Autodesk Inventor part; units mm, degrees
ref_plane "hh_XY" through (0, 3.175, 0) normal (0, 0, 1) x (1, 0, 0)
ref_plane "hh_YZ" through (0, 3.175, 0) normal (1, 0, 0) x (0, 1, 0)
ref_plane "hh_ZX" through (0, 3.175, 0) normal (0, 1, 0) x (0, 0, 1)
sketch "Sketch_1" plane through (0, 0, 0) normal (0, 0, 1) x (1, 0, 0)
  line L0 (6.35, 0) -> (0, 0)
  line L1 (0, 0) -> (0, 2.634)
  line L2 (0, 2.634) -> (0.541, 3.175)
  line L3 (0.541, 3.175) -> (6.35, 3.175)
  line L4 (6.35, 3.175) -> (6.35, 0)
  line L5 (6.35, 0) -> (0, 0)
revolve "Revolution1" add sketch "Sketch_1" angle 360 about axis through (6.35, 0, 0) along (1, 0, 0)
thread "Thread1"
sketch "Sketch_3" plane through (0, 0, 0) normal (0, 0, 1) x (1, 0, 0)
  line L0 (13.2715, 0) -> (6.35, 0)
  line L1 (6.35, 0) -> (6.35, 4.0513)
  line L2 (6.35, 4.0513) -> (6.858, 4.5593)
  line L3 (6.858, 4.5593) -> (9.398, 4.5593)
  line L4 (9.398, 4.5593) -> (9.398, 3.5242)
  line L5 (9.398, 3.5242) -> (9.9568, 3.5242)
  line L6 (9.9568, 3.5242) -> (10.5156, 4.0831)
  line L7 (10.5156, 4.0831) -> (12.7635, 4.0831)
  line L8 (12.7635, 4.0831) -> (13.2715, 3.5751)
  line L9 (13.2715, 3.5751) -> (13.2715, 0)
  line L10 (13.2715, 0) -> (6.35, 0)
revolve "Revolution2" add sketch "Sketch_3" angle 360 about axis through (13.2715, 0, 0) along (1, 0, 0)
sketch "Sketch_4" plane through (0, 0, 0) normal (0, 0, 1) x (1, 0, 0)
  line L0 (15.875, 0) -> (13.2715, 0)
  line L1 (13.2715, 0) -> (13.2715, 2.9845)
  line L2 (13.2715, 2.9845) -> (15.367, 2.9845)
  line L3 (15.367, 2.9845) -> (15.875, 2.4765)
  line L4 (15.875, 2.4765) -> (15.875, 0)
  line L5 (15.875, 0) -> (13.2715, 0)
revolve "Revolution3" add sketch "Sketch_4" angle 360 about axis through (15.875, 0, 0) along (1, 0, 0)
sketch "Sketch4" plane through (0, 0, 0) normal (-1, 0, 0) x (0, 0, 1)
  point P0 (0, 0)
hole "Hole1" at (0, 0, 0) direction (1, 0, 0) diameter 3.2512 depth 15.875 countersink diameter 4.0132 countersink angle 90
sketch "Sketch_47" plane through (0, 0, 0) normal (0, 0, 1) x (1, 0, 0)
  line L0 (9.9568, 0) -> (9.398, 0)
  line L1 (9.398, 4.0431) -> (9.398, 3.2702)
  line L2 (9.398, 3.2702) -> (9.9568, 3.2702)
  line L3 (9.9568, 3.2702) -> (9.9568, 3.5242)
  line L4 (9.9568, 3.5242) -> (9.6774, 3.5242)
  line L5 (9.6774, 3.5242) -> (9.5118, 3.6899)
  arc A0 (9.5118, 3.8695) -> (9.5118, 3.6899) centre (9.6016, 3.7797) ccw
  line L6 (9.5118, 3.8695) -> (10.1174, 4.4751)
  line L7 (10.1174, 4.4751) -> (10.1174, 4.5593)
  line L8 (10.1174, 4.5593) -> (9.9142, 4.5593)
  line L9 (9.9142, 4.5593) -> (9.398, 4.0431)
revolve "Revolution4" add sketch "Sketch_47" angle 360 about axis through (9.9568, 0, 0) along (1, 0, 0)
ref_plane "hh_XY" through (0, 3.175, 0) normal (0, 0, 1) x (1, 0, 0)
ref_plane "hh_YZ" through (0, 3.175, 0) normal (1, 0, 0) x (0, 1, 0)
ref_plane "hh_ZX" through (0, 3.175, 0) normal (0, 1, 0) x (0, 0, 1)
ref_plane "rod_guide_XY" through (0, 0, 0) normal (1, 0, 0) x (0, 0, -1)
ref_plane "rod_guide_YZ" through (0, 0, 0) normal (0, 0, -1) x (0, 1, 0)
ref_plane "rod_guide_ZX" through (0, 0, 0) normal (0, 1, 0) x (1, 0, 0)
ref_plane "t1_XY" through (6.35, 0, 0) normal (1, 0, 0) x (0, 0, -1)
ref_plane "t1_YZ" through (6.35, 0, 0) normal (0, 0, -1) x (0, 1, 0)
ref_plane "t1_ZX" through (6.35, 0, 0) normal (0, 1, 0) x (1, 0, 0)
ref_plane "t111_XY" through (6.35, 0, 0) normal (1, 0, 0) x (0, 0, -1)
ref_plane "t111_YZ" through (6.35, 0, 0) normal (0, 0, -1) x (0, 1, 0)
ref_plane "t111_ZX" through (6.35, 0, 0) normal (0, 1, 0) x (1, 0, 0)
ref_plane "to_foot_bracket_XY" through (6.35, 0, 0) normal (1, 0, 0) x (0, 0, -1)
ref_plane "to_foot_bracket_YZ" through (6.35, 0, 0) normal (0, 0, -1) x (0, 1, 0)
ref_plane "to_foot_bracket_ZX" through (6.35, 0, 0) normal (0, 1, 0) x (1, 0, 0)
ref_plane "to_nut_XY" through (6.35, 0, 0) normal (1, 0, 0) x (0, 0, -1)
ref_plane "to_nut_YZ" through (6.35, 0, 0) normal (0, 0, -1) x (0, 1, 0)
ref_plane "to_nut_ZX" through (6.35, 0, 0) normal (0, 1, 0) x (1, 0, 0)
ref_plane "to_rod_XY" through (0, 0, 0) normal (1, 0, 0) x (0, 0, -1)
ref_plane "to_rod_YZ" through (0, 0, 0) normal (0, 0, -1) x (0, 1, 0)
ref_plane "to_rod_ZX" through (0, 0, 0) normal (0, 1, 0) x (1, 0, 0)
ref_plane "to_screw_XY" through (6.35, 0, 0) normal (0, 1, 0) x (1, 0, 0)
ref_plane "to_screw_YZ" through (6.35, 0, 0) normal (1, 0, 0) x (0, 0, -1)
ref_plane "to_screw_ZX" through (6.35, 0, 0) normal (0, 0, -1) x (0, 1, 0)
ref_plane "to_trunnion_brackets_XY" through (0, 0, 0) normal (0, 1, 0) x (1, 0, 0)
ref_plane "to_trunnion_brackets_YZ" through (0, 0, 0) normal (1, 0, 0) x (0, 0, -1)
ref_plane "to_trunnion_brackets_ZX" through (0, 0, 0) normal (0, 0, -1) x (0, 1, 0)
ref_plane "to_trunnion_brackets1_XY" through (0, 6.35, 0) normal (0, 1, 0) x (1, 0, 0)
ref_plane "to_trunnion_brackets1_YZ" through (0, 6.35, 0) normal (1, 0, 0) x (0, 0, -1)
ref_plane "to_trunnion_brackets1_ZX" through (0, 6.35, 0) normal (0, 0, -1) x (0, 1, 0)
ref_plane "to_trunnion_brackets2_XY" through (0, -6.35, 0) normal (0, 1, 0) x (1, 0, 0)
ref_plane "to_trunnion_brackets2_YZ" through (0, -6.35, 0) normal (1, 0, 0) x (0, 0, -1)
ref_plane "to_trunnion_brackets2_ZX" through (0, -6.35, 0) normal (0, 0, -1) x (0, 1, 0)
ref_plane "to_tube_XY" through (9.9568, 0, 0) normal (1, 0, 0) x (0, 0, -1)
ref_plane "to_tube_YZ" through (9.9568, 0, 0) normal (0, 0, -1) x (0, 1, 0)
ref_plane "to_tube_ZX" through (9.9568, 0, 0) normal (0, 1, 0) x (1, 0, 0)
properties part number "007000-0_rod_guide"
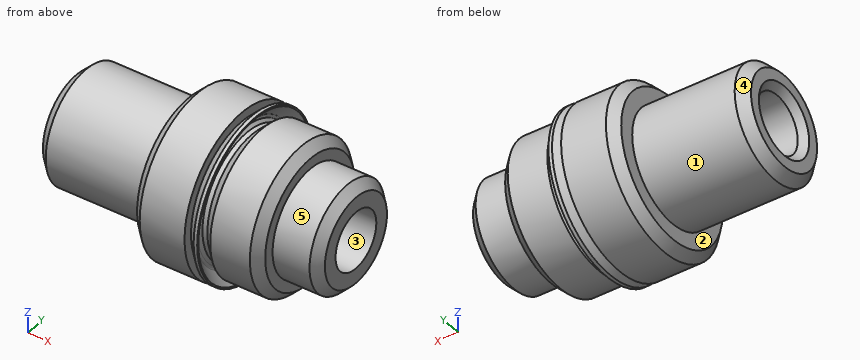
The model under review builds one solid part; all positions refer to its coordinate system, in mm. Face numbers are marked on the shaded views. A direction names the side the tool comes from. Give positions to 0.01 mm unless a question says otherwise; leave off trailing zeros. Write each loop counter-clockwise with the first axis right and the second up, starting at its lowest first coordinate (ties: lowest second). Pieces come first, ordered by that corner, then holes.
1. Tool access review of the marked faces 4 and 5: name each direction out of +Z, -Z, +X, -X, +Y, -Y from which nothing blocks a thin tool from reaching the whole face with its end or side.
2. Wall thickness on L1, parallel to X at y = 2, z = -2.75; L2, parallel to Y at x = 9.75, z = 1; L3, parallel to Z at x = 14, y = -0.75: over which ranges is each line inside the solid? List them lowest first.
3. For P1, Ø2, axis at y = 0, z = 0, coming from the +X side; P2, Ø3, axis at x = 4.5, z = 3, coming from the +Y side; P3, Ø1, axis at x = 14, z = 2.5, coming from the -Y side; P4, Ø1, axis at y = -0.5, z = 3, coming from the +X side, all flat-tipped, find the tip position at first contact; note any pin that passes through.
4. Draft analysis for pull direction Z (two halves, no side actions). For the marked faces 1, 2 and 3, state which applies: +Z half, -Z half, draft (parallel to the pull), parting line (faces both ways), or undercut.
5. Add section A-A, the plane x = 2.5. Write out the cut boundary in (y, z) (3 decimals), plus the area to 3 significant figures.
Worked answers:
1. face 4: -X
1. face 5: +X
2. L1: x = 6.35 to 13.27
2. L2: y = -4.28 to -3.98, -3.38 to -1.28, 1.28 to 3.38, 3.98 to 4.28
2. L3: z = -2.89 to -1.44, 1.44 to 2.89
3. P1: passes through
3. P2: stops at y = 2.8
3. P3: stops at y = -2.22
3. P4: stops at x = 15.81
4. face 1: parting line
4. face 2: draft
4. face 3: undercut
5. outline: circle Ø6.35 at (0, 0); hole circle Ø3.251 at (0, 0)
5. area: 23.4 mm2
